CAD build for the part. Positions are in the model's coordinates, mm. A direction names the side the tool comes from. Coordinates: 2 decimals unless noted, no trailing zeros. Order: outer loops, then holes, each group sorted by start corner. A loop starts at its lowest first (then second) coordinate and runs counter-clockwise, first axis right, second up. Notation, with made-up numbers: (14.25, -32) - (25.25, -32) arc R31 cw to (25.25, 6) - close; hole circle Ø9 at (23, 77). An arc over 180 degrees is marked (long way). Use one line per item in the form item = value.
```python
from build123d import *

# Parameters (mm, degrees)
F1_DEPTH = 50.8
F2_DEPTH = 25.4


with BuildPart() as f1:
    # F0 (on Top) → F1 (new body)
    with BuildSketch(Plane.XY):
        with BuildLine():
            ThreePointArc((3.650646, 41.4754), (-8.528173, 45.941043), (-21.498252, 45.734487))
            ThreePointArc((-21.498252, 45.734487), (-33.159754, 37.300433), (-38.737416, 24.033422))
            Line((-38.737416, 24.033422), (-38.737416, -10.444905))
            Line((-38.737416, -10.444905), (-38.737416, -14.095552))
            Line((-38.737416, -14.095552), (-38.737416, -41.069772))
            Line((-38.737416, -41.069772), (12.777264, -41.069772))
            Line((12.777264, -41.069772), (12.574449, -38.433194))
            Line((12.574449, -38.433194), (12.574449, -13.892737))
            Line((12.574449, -13.892737), (12.574449, 27.075628))
            ThreePointArc((12.574449, 27.075628), (9.485068, 35.12609), (3.650646, 41.4754))
        make_face()
    extrude(amount=F1_DEPTH)

    # F0 (on Top) → F2 (join)
    with BuildSketch(Plane.XY):
        with BuildLine():
            ThreePointArc((3.650646, 41.4754), (-8.528173, 45.941043), (-21.498252, 45.734487))
            ThreePointArc((-21.498252, 45.734487), (-33.159754, 37.300433), (-38.737416, 24.033422))
            Line((-38.737416, 24.033422), (-38.737416, -10.444905))
            Line((-38.737416, -10.444905), (-38.737416, -14.095552))
            Line((-38.737416, -14.095552), (-38.737416, -41.069772))
            Line((-38.737416, -41.069772), (12.777264, -41.069772))
            Line((12.777264, -41.069772), (12.574449, -38.433194))
            Line((12.574449, -38.433194), (12.574449, -13.892737))
            Line((12.574449, -13.892737), (12.574449, 27.075628))
            ThreePointArc((12.574449, 27.075628), (9.485068, 35.12609), (3.650646, 41.4754))
        make_face()
    extrude(amount=F2_DEPTH)


solid = f1.part
```
Item 1: Drill centre lines: line 1 (X direction, y = 20, z = 19); line 2 (X direction, y = 30, z = 35); line 3 (Y direction, x = -29, z = 30.5). Where is each one in solid material? Low to high. Write a range as [from, to].
Derived:
line_1 = [-38.74, 12.57]
line_2 = [-37.28, 11.85]
line_3 = [-41.07, 41.49]
Item 2: Cut at C-C, the plane y = 28. Write the cut outline in (x, z).
Derived:
outline = (-37.93, 0) - (12.39, 0) - (12.39, 50.8) - (-37.93, 50.8) - close
Item 3: Drop flat-ended pins along their axis: pin 1 (6 mm diameter, centred on y = -30.5, z = 21, fed in from +X); pin 2 (6 mm diameter, centred on y = 32.5, z = 36.5, fed in from -X); pin 3 (5 mm diameter, centred on x = -10.5, z = 41, fed in from +Y). Give the stop position or say it passes through.
Derived:
pin_1 = 12.57
pin_2 = -37.46
pin_3 = 46.41
Item 4: Cut at A-A, the plane z = 34.5. Write the cut outline in (x, y).
Derived:
outline = (-38.74, -41.07) - (12.78, -41.07) - (12.57, -38.43) - (12.57, 27.08) arc R23.02 ccw to (3.65, 41.48) arc R35.51 ccw to (-21.5, 45.73) arc R26.66 ccw to (-38.74, 24.03) - close
Item 5: 3-axis set-ups, long thin cutter, end or side, ignore diameter. For faces 1 (the face through (12.574, -6, 25)), 2 (the face through (-33, 37.5, 25)): which of +Z, -Z, +X, -X, +Y, -Y reach the whole face in a straight line?
Derived:
face_1 = +Z, -Z, +X, +Y
face_2 = +Z, -Z, -X, +Y
Item 6: Cut at B-B, the plane x = -0.5. Write the cut outline in (y, z), plus the area to 3 significant figures.
Derived:
outline = (-41.07, 0) - (43.58, 0) - (43.58, 50.8) - (-41.07, 50.8) - close
area = 4,300 mm²
